Here's how the part is built. I have some questions about the finished solid (model axes, mm). Face numbers are marked on the shaded views. A direction names the side the tool comes from. Coordinates: 2 decimals unless noted, no trailing zeros. Write each loop counter-clockwise with the first axis right and the second up, starting at its lowest first coordinate (ties: lowest second). Pieces come first, ordered by that corner, then holes.
from build123d import *

# Parameters (mm, degrees)
F0_W     = 30
F0_H     = 10
F0_W_2   = 15
F1_DEPTH = 20
F3_D     = 6
F4_D     = 12
F4_DEPTH = 4
F4_TIP   = 3.6051637142
F5_R     = 5
F6_R     = 15


with BuildPart() as f1:
    # F0 (on Top) → F1 (new body)
    with BuildSketch(Plane.XY):
        with Locations((-105, 0)):
            Rectangle(F0_W, F0_H)
        with Locations((-82.5, 0)):
            Rectangle(F0_W_2, F0_H)
        Polygon((-75, -5), (-90, -5), (-75, -52.6969600708), (75, -52.6969600708), (90, -5), (75, -5), (65, -41.5166201833), (-65, -41.5166201833), align=None)
        with Locations((82.5, 0)):
            Rectangle(F0_W_2, F0_H)
        with Locations((105, 0)):
            Rectangle(F0_W, F0_H)
    extrude(amount=F1_DEPTH)

    # F3 (through all)
    with Locations(Plane.XZ.offset(5)):
        with Locations((-112, 10), (-98, 10), (98, 10), (112, 10)):
            Hole(F3_D / 2)

    # F4
    with Locations(Plane.XZ.offset(5)):
        with Locations((-112, 10), (-98, 10), (98, 10), (112, 10)):
            Hole(F4_D / 2, depth=F4_DEPTH)
            with Locations((0, 0, -(F4_DEPTH + F4_TIP / 2))):  # 118° drill point
                Cone(0, F4_D / 2, F4_TIP, mode=Mode.SUBTRACT)

    # F5
    f5_edges = [f1.edges().sort_by_distance(p)[0] for p in [
        (-120, 0, 20),
        (-120, 0, 0),
        (120, 0, 20),
        (120, 0, 0),
    ]]
    fillet(f5_edges, radius=F5_R)

    # F6
    f6_edges = [f1.edges().sort_by_distance(p)[0] for p in [
        (-75, -52.69696, 10),
        (75, -52.69696, 10),
        (-65, -41.51662, 10),
        (65, -41.51662, 10),
        (-75, -5, 10),
        (75, -5, 10),
    ]]
    fillet(f6_edges, radius=F6_R)


solid = f1.part
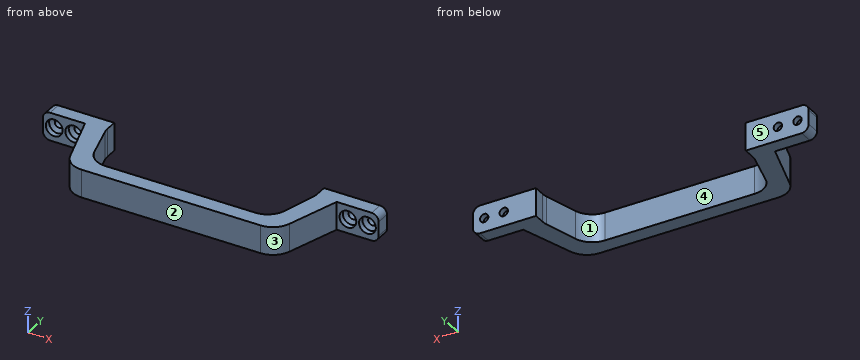
1. Thinking about a two-plate mould opening in X: for the marked faces 1, 2 and 3, which applies, pulls with the +X half, pulls with the -X half, needs draft (parallel to the pull), parting line crosses it, or undercut?
2. I want a section at B-B (y = -16). List the corners of the cut face in (x, z) for me, then the cut area to 3 significant figures.
3. I want a section at D-D (y = -36). List the corners of the cut face in (x, z) for me.
4. On a 3-axis mill with a long thin cutter (end or side, diameter ignored), from which of +Z, -Z, +X, -X, +Y, -Y can I reach the whole of each face in a straight line? I mean the marked faces 4 and 5. Say none if no direction works.
5. I want a section at A-A (x = 98). List the corners of the cut face in (y, z) for me.
6. I want a section at C-C (x = 51). List the corners of the cut face in (y, z) for me, then the cut area to 3 significant figures.
7. If I drill on line 1 (X direction, y = -3.3, z = 10); line 2 (X direction, y = 3.95, z = 10); line 3 (Z direction, x = 112, y = -2), over which ranges is the centre line in solid material (lowest first)?
8. For pin 1 Ø3 at (y, z) = (-41.5, 12) entering from +X; pin 2 Ø7 at (x, z) = (98, 10) entering from -Y; pin 3 Ø10 at (x, z) = (107.5, 5) entering from -Y, each with a flat end and sliding along its axis, tell me the tip position at first contact or that it passes through.
Response values:
1. face 1: undercut
1. face 2: needs draft
1. face 3: pulls with the +X half
2. outline: (-86.54, 0) - (-71.99, 0) - (-71.99, 20) - (-86.54, 20) - close; (71.99, 0) - (86.54, 0) - (86.54, 20) - (71.99, 20) - close
2. area: 582 mm2
3. outline: (-80.25, 0) - (-65.18, 0) - (-65.18, 20) - (-80.25, 20) - close; (65.18, 0) - (80.25, 0) - (80.25, 20) - (65.18, 20) - close
4. face 4: +Z, -Z, +Y
4. face 5: +Z, -Z, +X, -X, +Y
5. outline: (-5, 0) - (5, 0) - (5, 7) - (0.8, 7) - (-1, 4) - (-5, 4) - close; (-5, 16) - (-1, 16) - (0.8, 13) - (5, 13) - (5, 20) - (-5, 20) - close
6. outline: (-52.7, 0) - (-41.52, 0) - (-41.52, 20) - (-52.7, 20) - close
6. area: 224 mm2
7. line 1: x = -120 to -118, -106 to -104, -92 to -75, 75 to 92, 104 to 106, 118 to 120
7. line 2: x = -120 to -115, -109 to -101, -95 to -75, 75 to 95, 101 to 109, 115 to 120
7. line 3: z = 0 to 4, 16 to 20
8. pin 1: stops at x = 78.99
8. pin 2: stops at y = 0.5
8. pin 3: stops at y = -5
